from build123d import *

# Parameters (mm, degrees)
ESTRUSIONE_ESTRUSIONE1_DEPTH = 190


with BuildPart() as part:
    # Schizzo2 → Estrusione-Estrusione1 (new body)
    with BuildSketch(Plane(origin=(0, 0, 0), x_dir=(1, 0, 0), z_dir=(0, 1, 0))):
        Polygon((415.547769121, 607.865337729), (331.895708168, 607.865337729), (322.188097577, 607.865337729), (316.547769121, 607.865337729), (316.547769121, 600.865337729), (322.188097577, 600.865337729), (322.188097577, 604.865337729), (331.948189583, 604.865337729), (331.948189583, 585.865337729), (322.188097577, 585.865337729), (322.188097577, 589.865337729), (316.547769121, 589.865337729), (316.547769121, 582.865337729), (415.547769121, 582.865337729), align=None)
    estrusione_estrusione1 = extrude(amount=ESTRUSIONE_ESTRUSIONE1_DEPTH)

    # Specchia1: Estrusione-Estrusione1 across plane
    add(estrusione_estrusione1.mirror(Plane(origin=(415.547769121, 190, 0), x_dir=(0, 0, 1), z_dir=(1, 0, 0))))


solid = part.part
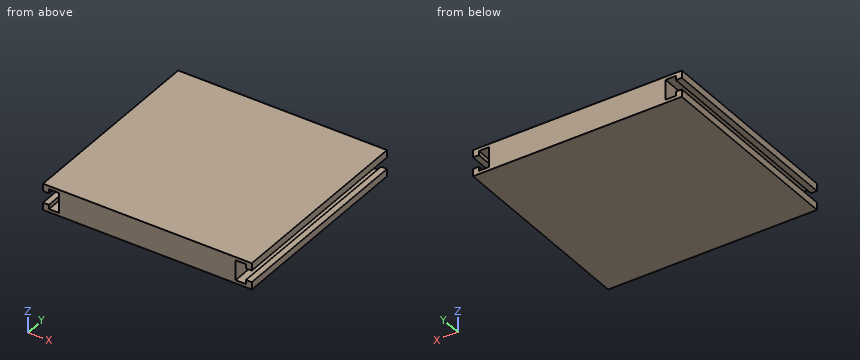
Read the model definition and answer for the solid it produces. Units are mm, in the model's axes. Give positions to 0.01 mm unless a question says otherwise; leave off trailing zeros. Write each loop counter-clockwise with the first axis right and the second up, starting at its lowest first coordinate (ties: lowest second). Pieces come first, ordered by that corner, then holes. Notation, with made-up numbers: (2.25, -1) - (23.25, -1) arc R25 cw to (23.25, 14) - close; hole circle Ø6 at (-15, -1). An arc over 180 degrees is marked (long way). Return JSON: item names as keys, results as strings.
Q1. Given P1, Ø3, axis at y = 92, z = -592, coming from the -X side; P2, Ø1.5, axis at y = 69, z = -598, coming from the +X side, each flat-ended and moving along its own axis, determine where each tip first touches the part or whether it passes through.
Reply:
{"P1": "x = 331.95", "P2": "x = 499.15"}
Q2. A cutting plane is placed at A-A, the plane y = 54. Determine the outline of the cut face in (x, z).
Reply:
{"outline": "(316.55, -607.87) - (514.55, -607.87) - (514.55, -600.87) - (508.91, -600.87) - (508.91, -604.87) - (499.15, -604.87) - (499.15, -585.87) - (508.91, -585.87) - (508.91, -589.87) - (514.55, -589.87) - (514.55, -582.87) - (316.55, -582.87) - (316.55, -589.87) - (322.19, -589.87) - (322.19, -585.87) - (331.95, -585.87) - (331.95, -604.87) - (322.19, -604.87) - (322.19, -600.87) - (316.55, -600.87) - close"}
Q3. Consider line 1 along X through (y, z) = (25, -587.25); line 2 along X through (y, z) = (132, -595). Determine where each line is inside the solid, lowest interval first. Write a range as [from, to].
Reply:
{"line 1": "[316.55, 322.19], [331.95, 499.15], [508.91, 514.55]", "line 2": "[331.95, 499.15]"}
Q4. A cutting plane is placed at B-B, the plane z = -594.5. Determine the outline of the cut face in (x, y).
Reply:
{"outline": "(331.95, 0) - (499.15, 0) - (499.15, 190) - (331.95, 190) - close"}
